Build history of the part. All positions in model axes, mm. Give positions to 0.01 mm unless a question says otherwise; leave off trailing zeros. Write each loop counter-clockwise with the first axis right and the second up, starting at its lowest first coordinate (ties: lowest second). Pieces come first, ordered by that corner, then holes. Notation, with made-up numbers: (-2, 10.25) -> (17, 10.25) arc R27 cw to (17, 43.25) -> close; hole circle Ø2 at (-12, -38). An arc over 180 degrees is marked (long way). Put each result on its own line as item: value.
from build123d import *

# Parameters (mm, degrees)
PLAT_W                          = 30
PLAT_H                          = 5
EL_MENT_M_CANO_SOUD_1_DEPTH     = 1066
DIAM_TRE_DU_PER_AGE_13_0_13_1_D = 13
R_P_TITION_LIN_AIRE2_COUNT      = 3
R_P_TITION_LIN_AIRE2_PITCH      = 473


with BuildPart() as part:
    # plat → Elément mécano-soudé1 (new body)
    with BuildSketch(Plane.YZ.offset(-533)):
        Rectangle(PLAT_W, PLAT_H)
    extrude(amount=EL_MENT_M_CANO_SOUD_1_DEPTH)

    # Diamètre du perçage Ø13.0 (13)1 (through all)
    with Locations(Plane(origin=(0, 0, -2.5), x_dir=(-1, 0, 0), z_dir=(0, 0, -1))):
        with Locations((473, 0)):
            diam_tre_du_per_age_13_0_13_1 = Hole(DIAM_TRE_DU_PER_AGE_13_0_13_1_D / 2)

    # Répétition linéaire2: Diamètre du perçage Ø13.0 (13)1 ×3
    with Locations(*[(i * R_P_TITION_LIN_AIRE2_PITCH, 0, 0) for i in range(1, R_P_TITION_LIN_AIRE2_COUNT)]):
        add(diam_tre_du_per_age_13_0_13_1, mode=Mode.SUBTRACT)


solid = part.part
1) Wall check: L1, parallel to Y at x = 0, z = 1.45; L2, parallel to X at y = -5.5, z = 1.8; L3, parallel to X at y = -3.5, z = 1.6. Give the ranges that are in metal, low to high.
Filled sheet:
L1: -15 to -6.5, 6.5 to 15
L2: -533 to -476.46, -469.54 to -3.46, 3.46 to 469.54, 476.46 to 533
L3: -533 to -478.48, -467.52 to -5.48, 5.48 to 467.52, 478.48 to 533
2) Slice it at A-A (y = 0). Write the cut outline in (x, z), plus the area to 4 significant figures.
Filled sheet:
outline: (-533, -2.5) -> (-479.5, -2.5) -> (-479.5, 2.5) -> (-533, 2.5) -> close; (-466.5, -2.5) -> (-6.5, -2.5) -> (-6.5, 2.5) -> (-466.5, 2.5) -> close; (6.5, -2.5) -> (466.5, -2.5) -> (466.5, 2.5) -> (6.5, 2.5) -> close; (479.5, -2.5) -> (533, -2.5) -> (533, 2.5) -> (479.5, 2.5) -> close
area: 5,135 mm2
3) Pin check, flat tip, straight feed: pin 1 (10.5 mm diameter, centred on x = 0, y = 0, fed in from -Z). Stop position of the tip, or through.
Filled sheet:
pin 1: through
